from build123d import *

# Parameters (mm, degrees)
F0_W     = 1.8
F0_H     = 1.8
F0_W_2   = 1.475
F0_H_2   = 1.475
F1_DEPTH = 31.5


with BuildPart() as f1:
    # F0 (on Front) → F1 (new body)
    with BuildSketch(Plane.XZ):
        Rectangle(F0_W, F0_H)
        with Locations((-1.6375, 0)):
            Rectangle(F0_W_2, F0_H)
        with Locations((0, 1.6375)):
            Rectangle(F0_W, F0_H_2)
        with Locations((0, -1.6375)):
            Rectangle(F0_W, F0_H_2)
        with Locations((1.6375, 0)):
            Rectangle(F0_W_2, F0_H)
    extrude(amount=F1_DEPTH)


solid = f1.part
The listing builds one solid part. Answer for the finished solid, in the listing's coordinates (mm). A direction names the side the tool comes from. Coordinates: 2 decimals unless noted, no trailing zeros. Loops run counter-clockwise (first coordinate to the right, second up) from the corner with the lowest first, then second, coordinate; pieces in that order, holes last.
1) Find section B-B on x = -1.75. Write down the section's boundary in (y, z), then the cut area to 3 significant figures.
2) Find section C-C on z = 2. Write down the section's boundary in (x, y).
3) Flat-ended cylindrical pins translate along their axes: pin 1 Ø1.6 at (y, z) = (-16.5, 1.5) entering from -X (3 decimals); pin 2 Ø0.7 at (y, z) = (-10.5, -1.5) entering from +X; pin 3 Ø1.2 at (x, y) = (2, -11.5) entering from +Z; pin 4 Ø0.7 at (y, z) = (-10.5, -1.5) entering from -X. Find the tip coordinate at first contact, or state that the pin passes through.
4) Find section A-A on y = -20.5. Write down the section's boundary in (x, z) (3 decimals).
5) A tool of negligible diameter and unlimited length cuts with its end or side. For faces 1 (the face through (2, -16, 0.9)), 2 (the face through (2, -16, -0.9)), 3 (the face through (-2, -16, -0.9)), 4 (the face through (-2, -16, 0.9)), from which of +Z, -Z, +X, -X, +Y, -Y can it reach the whole face along a straight path? Write none if from no direction.
6) Find the intervals of material crossed by L1, parallel to Z at x = -1.7, y = -13, in increasing order.
Values:
1. outline: (-31.5, -0.9) - (0, -0.9) - (0, 0.9) - (-31.5, 0.9) - close
1. area: 56.7 mm2
2. outline: (-0.9, -31.5) - (0.9, -31.5) - (0.9, 0) - (-0.9, 0) - close
3. pin 1: stops at x = -2.375
3. pin 2: stops at x = 0.9
3. pin 3: stops at z = 0.9
3. pin 4: stops at x = -0.9
4. outline: (-2.375, -0.9) - (-0.9, -0.9) - (-0.9, -2.375) - (0.9, -2.375) - (0.9, -0.9) - (2.375, -0.9) - (2.375, 0.9) - (0.9, 0.9) - (0.9, 2.375) - (-0.9, 2.375) - (-0.9, 0.9) - (-2.375, 0.9) - close
5. face 1: +Z, +X, +Y, -Y
5. face 2: -Z, +X, +Y, -Y
5. face 3: -Z, -X, +Y, -Y
5. face 4: +Z, -X, +Y, -Y
6. L1: z = -0.9 to 0.9
